from build123d import *

# Parameters (mm, degrees)
ESQUISSE2_R             = 2.5
ENL_V_MAT_EXTRU_1_DEPTH = 44.678427169
ESQUISSE3_W             = 2
ESQUISSE3_H             = 2.737754662
ENL_V_MAT_EXTRU_2_DEPTH = 52.408219187
ESQUISSE4_R             = 3
ENL_V_MAT_EXTRU_3_DEPTH = 20
CHANFREIN1_SIZE         = 0.5


with BuildPart() as part:
    # Esquisse1 → Révolution1 (revolve)
    with BuildSketch(Plane.XY, mode=Mode.PRIVATE) as r_volution1_sk:
        Polygon((-15, 4), (-15, 14), (-5, 14), (-5, 15), (0, 15), (0, 28.45), (17, 28.45), (17, 4), align=None)
    revolve(r_volution1_sk.sketch.rotate(Axis((-36.38001638, 0, 0), (1, 0, 0)), 90), axis=Axis((-36.38001638, 0, 0), (1, 0, 0)))

    # Esquisse2 → Enlèv. mat.-Extru.1 (cut, through all)
    with BuildSketch(Plane.ZY):
        with Locations((0, 23.75)):
            Circle(ESQUISSE2_R)
        with Locations((20.56810334, 11.875)):
            Circle(ESQUISSE2_R)
        with Locations((20.56810334, -11.875)):
            Circle(ESQUISSE2_R)
        with Locations((0, -23.75)):
            Circle(ESQUISSE2_R)
        with Locations((-20.56810334, -11.875)):
            Circle(ESQUISSE2_R)
        with Locations((-20.56810334, 11.875)):
            Circle(ESQUISSE2_R)
    extrude(amount=-ENL_V_MAT_EXTRU_1_DEPTH, mode=Mode.SUBTRACT)

    # Esquisse3 → Enlèv. mat.-Extru.2 (cut, through all)
    with BuildSketch(Plane.ZY.offset(15)):
        with Locations((0, 3.631122669)):
            Rectangle(ESQUISSE3_W, ESQUISSE3_H)
    extrude(amount=-ENL_V_MAT_EXTRU_2_DEPTH, mode=Mode.SUBTRACT)

    # Esquisse4 → Enlèv. mat.-Extru.3 (cut)
    with BuildSketch(Plane.XY):
        with Locations((-10, 0)):
            Circle(ESQUISSE4_R)
    extrude(amount=-ENL_V_MAT_EXTRU_3_DEPTH, mode=Mode.SUBTRACT)

    # Chanfrein1
    chanfrein1_edges = [part.edges().sort_by_distance(p)[0] for p in [
        (17, 0, -28.45),
        (0, 0, -28.45),
        (-5, 0, -15),
        (-15, 0, -14),
    ]]
    chamfer(chanfrein1_edges, length=CHANFREIN1_SIZE)


solid = part.part
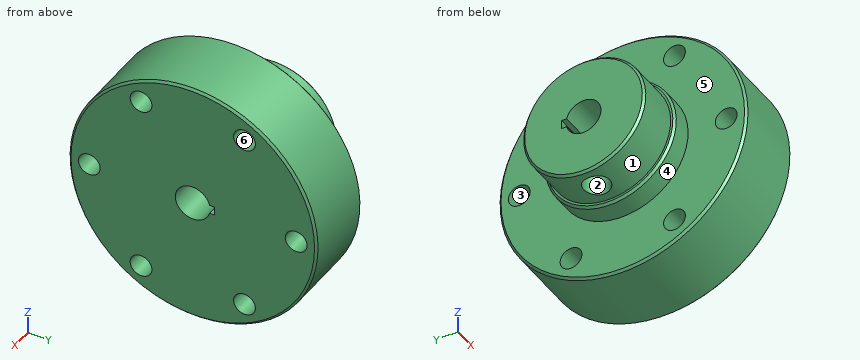
The listing builds one solid part. Answer for the finished solid, in the listing's coordinates (mm). Face numbers are marked on the shaded views. A direction names the side the tool comes from. Round coordinates to 2 decimals unless told otherwise and drop trailing zeros. Write each loop counter-clockwise with the first axis right and the second up, starting at its lowest first coordinate (ties: lowest second). Pieces come first, ordered by that corner, then holes. Notation, with made-up numbers: (-7, 58) - (3, 58) arc R21 ccw to (3, 95) - close; hole circle Ø10 at (-30, 52.25). An arc over 180 degrees is marked (long way). Use a Markdown table: item, result. Add a question column.
1. Consider line 1 (Y direction, x = 7.5, z = 0); line 2 (Z direction, x = 4.5, y = -13.5); line 3 (Y direction, x = 3.5, z = 21.5). Determine where each line is inside the solid, lowest interval first.
2. The part is cut by section C-C (x = 7). Write down the section's boundary in (y, z) (3 decimals).
3. Flat-ended cylindrical pins translate along their axes: P1, Ø10, axis at x = -0.5, z = -21, coming from the -Y side; P2, Ø3, axis at y = 11.88, z = 20.57, coming from the +X side; P3, Ø6, axis at x = -4, z = -4.5, coming from the -Y side; P4, Ø2, axis at x = -11.5, z = 0.5, coming from the +Y side. Find the tip coordinate at first contact, or state that the pin passes through.
4. For a pull along Y with two mould halves and no side action, classify the marked faces 4, 5 and 6 as +Y half, -Y half, draft (parallel to the pull), parting line (faces both ways), or undercut.
5. The part is cut by section A-A (z = 0). Give the number of separate pieces and of enclosed holes in the cut face, and give its area (3 significant figures).
6. The part is cut by section B-B (y = 0). Write down the section's boundary in (x, z).
7. The part is cut by section D-D (x = -8). Write down the section's boundary in (y, z), and give its area (3 significant figures).
8. A tool of negligible diameter and unlimited length cuts with its end or side. For the marked faces 1, 2 and 3, from which of +Z, -Z, +X, -X, +Y, -Y can it reach the whole face along a straight path? Write none if from no direction.
Reported:
| question | item | result |
|---|---|---|
| 1 | line 1 | -28.45 to -26.25, -21.25 to -4, 5 to 21.25, 26.25 to 28.45 |
| 1 | line 2 | -25.04 to -22.47, -18.67 to 18.67, 22.47 to 25.04 |
| 1 | line 3 | -18.63 to -14.19, -9.56 to 9.56, 14.19 to 18.63 |
| 2 | outline | circle Ø56.9 at (0, 0); hole circle Ø5 at (-23.75, 0); hole circle Ø5 at (-11.875, -20.568); hole circle Ø5 at (-11.875, 20.568); hole (3.873, -1) - (5, -1) - (5, 1) - (3.873, 1) arc R4 ccw (long way) to start; hole circle Ø5 at (11.875, -20.568); hole circle Ø5 at (11.875, 20.568); hole circle Ø5 at (23.75, 0) |
| 3 | P1 | y = -23.46 |
| 3 | P2 | through |
| 3 | P3 | y = -14.92 |
| 3 | P4 | y = 14 |
| 4 | face 4 | parting line |
| 4 | face 5 | draft |
| 4 | face 6 | undercut |
| 5 | separate pieces | 4 |
| 5 | enclosed holes | 0 |
| 5 | area | 938 mm^2 |
| 6 | outline | (-15, -13.5) - (-14.5, -14) - (-13, -14) - (-13, -4) - (-15, -4) - close; (-15, 4) - (17, 4) - (17, 27.95) - (16.5, 28.45) - (0.5, 28.45) - (0, 27.95) - (0, 15) - (-4.5, 15) - (-5, 14.5) - (-5, 14) - (-14.5, 14) - (-15, 13.5) - close; (-7, -14) - (-5, -14) - (-5, -14.5) - (-4.5, -15) - (0, -15) - (0, -27.95) - (0.5, -28.45) - (16.5, -28.45) - (17, -27.95) - (17, -4) - (-7, -4) - close |
| 7 | outline | (-2.24, -13.82) - (-2.24, -3.32) arc R4 cw (long way) to (3.87, 1) - (5, 1) - (5, -1) - (3.87, -1) arc R4 cw to (2.24, -3.32) - (2.24, -13.82) arc R14 ccw (long way) to start |
| 7 | area | 518 mm^2 |
| 8 | face 1 | -X |
| 8 | face 2 | -Z |
| 8 | face 3 | +X, -X |
